Autodesk Inventor part; units mm, degrees
ref_plane "YZ Plane" through (0, 0, 0) normal (1, 0, 0) x (0, 1, 0)
ref_plane "XZ Plane" through (0, 0, 0) normal (0, 1, 0) x (-1, 0, 0)
ref_plane "XY Plane" through (0, 0, 0) normal (0, 0, 1) x (1, 0, 0)
sketch "Sketch2" plane through (0, 0, 0) normal (0, 0, 1) x (1, 0, 0)
  line L0 (-4.7023, 28.2327) -> (-5.3373, 28.2327)
  line L1 (-5.3373, 28.2327) -> (-5.3373, 26.3277)
  line L2 (-4.7023, 26.3277) -> (-4.7023, 28.2327)
  line L3 (-5.3373, 26.3277) -> (-4.7023, 26.3277)
  arc A0 (-5.4629, 26.9627) -> (-6.3519, 26.0737) centre (-5.4629, 26.0737) ccw
  line L4 (-4.5766, 26.9627) -> (-5.4629, 26.9627)
  arc A1 (-3.6876, 26.0737) -> (-4.5766, 26.9627) centre (-4.5766, 26.0737) ccw
  line L5 (-3.6876, 15.1517) -> (-3.6876, 26.0737)
  arc A2 (-4.5766, 14.2627) -> (-3.6876, 15.1517) centre (-4.5766, 15.1517) ccw
  line L6 (-5.4629, 14.2627) -> (-4.5766, 14.2627)
  arc A3 (-6.3519, 15.1517) -> (-5.4629, 14.2627) centre (-5.4629, 15.1517) ccw
  line L7 (-6.3519, 26.0737) -> (-6.3519, 15.1517)
  line L8 (-6.3519, 14.2627) -> (-3.6876, 26.9627) construction
  line L9 (-3.6876, 14.2627) -> (-6.3519, 26.9627) construction
  line L10 (-5.3373, 26.3277) -> (-4.7023, 28.2327) construction
  line L11 (-4.7023, 26.3277) -> (-5.3373, 28.2327) construction
  circle A4 centre (-5.0198, 30.0107) radius 2.54
  circle A5 centre (-5.7772, 26.3881) radius 0.0635
  line L12 (-5.4629, 26.0737) -> (-6.0915, 26.7024) construction
  line L13 (-5.0198, 20.6127) -> (-3.948, 20.6127)
  line L14 (-3.948, 20.6127) -> (-5.0198, 20.6127)
  line L15 (-5.0198, 20.6127) -> (-5.0198, 22.4129)
  circle A6 centre (-4.2623, 26.3881) radius 0.0635
  circle A7 centre (-5.7772, 14.8374) radius 0.0635
  circle A8 centre (-4.2623, 14.8374) radius 0.0635
  point P0 (0, 0)
  point P1 (-5.3373, 26.9627)
  point P2 (-4.7023, 26.9627)
  point P3 (-4.7023, 27.4907)
  point P4 (-5.3373, 27.4907)
  dimension "d7" = 5.08
  dimension "d8" = 3.048
  dimension "d9" = 0.127
  dimension "d10" = 0.4445
extrude "Extrusion1" add sketch "Sketch2" along normal mid plane 0.254
properties material "ABS Plastic"
Can you work these out from the model? Positions are in its coordinate system, mm. Coordinates: 2 decimals unless noted, no trailing zeros. Order: outer loops, then holes, each group sorted by start corner. A loop starts at its lowest first (then second) coordinate and runs counter-clockwise, first axis right, second up. Notation, with made-up numbers: M 13.25,68.25 L 33.25,68.25 A26 cw 33.25,93.25 Z; hole C 50.25,24 d3. An arc over 180 degrees is marked long. Answer as CSV lines item,"result".
(1) Please list where these lines run through material, in increasing order: L1, parallel to X at y = 18, z = -0.05; L2, parallel to Y at x = -5.4, z = 0.05; L3, parallel to X at y = 28.25, z = 0.05.
Geometry check:
L1,"-6.35 to -3.69"
L2,"14.26 to 26.96, 27.5 to 32.52"
L3,"-6.85 to -3.19"
(2) Suppose I cut it at C-C on x = -7.1. Please give me the cut outline in (y, z), plus the area to 3 significant figures.
Geometry check:
outline,"M 28.55,-0.13 L 31.47,-0.13 L 31.47,0.13 L 28.55,0.13 Z"
area,"0.740 mm^2"
(3) Suppose I cut it at A-A on z = 0. Please give me the cut outline in (x, y), plus the area to 3 significant figures.
Geometry check:
outline,"M -6.35,15.15 A0.89 ccw -5.46,14.26 L -4.58,14.26 A0.89 ccw -3.69,15.15 L -3.69,26.07 A0.89 ccw -4.58,26.96 L -4.7,26.96 L -4.7,27.49 A2.54 ccw long -5.34,27.49 L -5.34,26.96 L -5.46,26.96 A0.89 ccw -6.35,26.07 Z; hole C -5.78,14.84 d0.13; hole C -5.78,26.39 d0.13; hole C -4.26,14.84 d0.13; hole C -4.26,26.39 d0.13"
area,"53.7 mm^2"
(4) Suppose I cut it at B-B on y = 20. Please give me the cut outline in (x, z), plus the area to 3 significant figures.
Geometry check:
outline,"M -6.35,-0.13 L -3.69,-0.13 L -3.69,0.13 L -6.35,0.13 Z"
area,"0.677 mm^2"
